Can you work these out from the model? Positions are in its coordinate system, mm. A direction names the side the tool comes from. Give positions to 0.01 mm unless a question says otherwise; leave off trailing zeros. Write each loop counter-clockwise with the first axis right and the second up, starting at its lowest first coordinate (ties: lowest second). Pieces come first, ordered by that corner, then holes.
```python
from build123d import *

# Parameters (mm, degrees)
SKETCH1_R           = 1.25
BOSS_EXTRUDE1_DEPTH = 9
SKETCH2_R           = 2.5
BOSS_EXTRUDE2_DEPTH = 2
SKETCH3_W           = 6
SKETCH3_H           = 2.5
BOSS_EXTRUDE3_DEPTH = 2


with BuildPart() as part:
    # Sketch1 → Boss-Extrude1 (new, symmetric)
    with BuildSketch(Plane.XY):
        Circle(SKETCH1_R)
    extrude(amount=BOSS_EXTRUDE1_DEPTH, both=True)

    # Sketch2 → Boss-Extrude2 (add)
    with BuildSketch(Plane.XY.offset(9)):
        Circle(SKETCH2_R)
    extrude(amount=BOSS_EXTRUDE2_DEPTH)

    # Sketch3 → Boss-Extrude3 (add)
    with BuildSketch(Plane(origin=(0, 0, -9), x_dir=(-1, 0, 0), z_dir=(0, 0, -1))):
        Rectangle(SKETCH3_W, SKETCH3_H)
    extrude(amount=BOSS_EXTRUDE3_DEPTH)


solid = part.part
```
1) If we mould it in two halves opening along Z, with no side actions, what happens to faces 6 (the face through (0, 0, -11)), 7 (the face through (-2, 0, -9)), 8 (the face through (0, -1.25, -10))? For each: +Z half, -Z half, draft (parallel to the pull), parting line (faces both ways), or undercut.
Values follow:
face 6: -Z half
face 7: undercut
face 8: draft
2) Please list where these lines run through material, in increasing order: L1, parallel to Z at x = 1.4, y = 0.45; L2, parallel to Z at x = 1.1, y = -1.3; L3, parallel to Y at x = 0.1, z = -5.
Values follow:
L1: z = -11 to -9, 9 to 11
L2: z = 9 to 11
L3: y = -1.25 to 1.25
3) Suppose I cut it at C-C on z = 3.5. Write out the boundary of the cut face in (x, y).
Values follow:
outline: circle Ø2.5 at (0, 0)
4) Suppose I cut it at A-A on y = 0. Write out the boundary of the cut face in (x, z), plus the area to 3 significant figures.
Values follow:
outline: (-3, -11) - (3, -11) - (3, -9) - (1.25, -9) - (1.25, 9) - (2.5, 9) - (2.5, 11) - (-2.5, 11) - (-2.5, 9) - (-1.25, 9) - (-1.25, -9) - (-3, -9) - close
area: 67.0 mm2
5) For pin 1 Ø1.5 at (y, z) = (-1.5, -3) entering from -X; pin 2 Ø2 at (x, z) = (1, -10) entering from -Y; pin 3 Ø2 at (x, z) = (1, -7.5) entering from +Y, each with a flat end and sliding along its axis, tell me the tip position at first contact or that it passes through.
Values follow:
pin 1: stops at x = -1
pin 2: stops at y = -1.25
pin 3: stops at y = 1.25
6) Suppose I cut it at D-D on y = 1.5. Write out the boundary of the cut face in (x, z).
Values follow:
outline: (-2, 9) - (2, 9) - (2, 11) - (-2, 11) - close
7) For faces 1 (the face through (0, 0, 11)), 2 (the face through (-1, -1, 9)), 3 (the face through (-0.54, -2.44, 9.99)), 4 (the face through (0, 1.25, -10)), 5 (the face through (-3, 0, -10)), which set-ups out of +Z, -Z, +X, -X, +Y, -Y let a thin tool reach every point of the face, with its end or its side?
Values follow:
face 1: +Z, +X, -X, +Y, -Y
face 2: none
face 3: +Z
face 4: -Z, +X, -X, +Y
face 5: +Z, -Z, -X, +Y, -Y
8) Suppose I cut it at B-B on x = -0.5. Write out the boundary of the cut face in (y, z).
Values follow:
outline: (-2.45, 9) - (-1.15, 9) - (-1.15, -9) - (-1.25, -9) - (-1.25, -11) - (1.25, -11) - (1.25, -9) - (1.15, -9) - (1.15, 9) - (2.45, 9) - (2.45, 11) - (-2.45, 11) - close
